Could you check a few things on this model? Use its own coordinates, in mm. A direction names the side the tool comes from. Round coordinates to 2 decimals unless told otherwise and drop trailing zeros. Loops run counter-clockwise (first coordinate to the right, second up) from the corner with the lowest first, then second, coordinate; pieces in that order, holes last. Notation, with made-up numbers: (23.25, -6.75) -> (58.25, -6.75) arc R24 ccw to (58.25, 22.25) -> close; hole circle Ø3 at (-27, -7). An arc over 180 degrees is marked (long way). One line per item, written item: value.
```python
from build123d import *

# Parameters (mm, degrees)
EXTRUDE_1_DEPTH          = 52
FILLET_1_R               = 5
CUT_EXTRUDE_1_DEPTH      = 10
CUT_EXTRUDE_1_DEPTH_BACK = 10
SKETCH_2_R               = 1.5
CUT_EXTRUDE_2_DEPTH      = 10
CUT_EXTRUDE_2_DEPTH_BACK = 1.5


with BuildPart() as part:
    # Эскиз1 → Бобышка-Вытянуть1 (new body)
    with BuildSketch(Plane(origin=(0, 0, 0), x_dir=(1, 0, 0), z_dir=(0, 1, 0))):
        Polygon((-17.5, -4.485282754), (-17.5, -8.485282754), (-6, -8.485282754), (-6, 4.485282754), (6, 4.485282754), (6, -8.485282754), (17.5, -8.485282754), (17.5, -4.485282754), (10, -4.485282754), (10, 8.485282754), (-10, 8.485282754), (-10, -4.485282754), align=None)
    extrude(amount=EXTRUDE_1_DEPTH)

    # Скругление1
    fillet_1_edges = [part.edges().sort_by_distance(p)[0] for p in [
        (-10, 26, 4.485282754),
        (-10, 26, -8.485282754),
        (10, 26, -8.485282754),
        (10, 26, 4.485282754),
    ]]
    fillet(fillet_1_edges, radius=FILLET_1_R)

    # Эскиз2 → Вырез-Вытянуть1 (cut, two sides: drawn at the far end of the back side and taken through both)
    with BuildSketch(Plane(origin=(0, 0, 4.485282754), x_dir=(-1, 0, 0), z_dir=(0, 0, -1)).offset(-CUT_EXTRUDE_1_DEPTH_BACK)):
        with Locations(Location((13.75, 41.6, 0), (0, 0, 33.557309762))):
            Circle(SKETCH_2_R)
        with Locations(Location((13.75, 31.6, 0), (0, 0, 33.557309762))):
            Circle(SKETCH_2_R)
        with Locations(Location((13.75, 21.6, 0), (0, 0, 33.557309762))):
            Circle(SKETCH_2_R)
        with Locations(Location((13.75, 11.6, 0), (0, 0, 33.557309762))):
            Circle(SKETCH_2_R)
        with Locations(Location((-13.75, 41.6, 0), (0, 0, 213.557309762))):
            Circle(SKETCH_2_R)
        with Locations(Location((-13.75, 31.6, 0), (0, 0, 146.442690238))):
            Circle(SKETCH_2_R)
        with Locations(Location((-13.75, 21.6, 0), (0, 0, 146.442690238))):
            Circle(SKETCH_2_R)
        with Locations(Location((-13.75, 11.6, 0), (0, 0, 146.442690238))):
            Circle(SKETCH_2_R)
    extrude(amount=CUT_EXTRUDE_1_DEPTH + CUT_EXTRUDE_1_DEPTH_BACK, mode=Mode.SUBTRACT)

    # Эскиз3 → Вырез-Вытянуть2 (cut, two sides: drawn at the far end of the back side and taken through both)
    with BuildSketch(Plane(origin=(0, 0, 4.485282754), x_dir=(-1, 0, 0), z_dir=(0, 0, -1)).offset(-CUT_EXTRUDE_2_DEPTH_BACK)):
        Polygon((13.75, 38.424573519), (16.5, 40.01228676), (16.5, 43.18771324), (13.75, 44.775426481), (11, 43.18771324), (11, 40.01228676), align=None)
        Polygon((-11, 40.01228676), (-13.75, 38.424573519), (-16.5, 40.01228676), (-16.5, 43.18771324), (-13.75, 44.775426481), (-11, 43.18771324), align=None)
        Polygon((13.75, 28.424573519), (16.5, 30.01228676), (16.5, 33.18771324), (13.75, 34.775426481), (11, 33.18771324), (11, 30.01228676), align=None)
        Polygon((-11, 30.01228676), (-13.75, 28.424573519), (-16.5, 30.01228676), (-16.5, 33.18771324), (-13.75, 34.775426481), (-11, 33.18771324), align=None)
        Polygon((13.75, 18.424573519), (16.5, 20.01228676), (16.5, 23.18771324), (13.75, 24.775426481), (11, 23.18771324), (11, 20.01228676), align=None)
        Polygon((-11, 20.01228676), (-13.75, 18.424573519), (-16.5, 20.01228676), (-16.5, 23.18771324), (-13.75, 24.775426481), (-11, 23.18771324), align=None)
        Polygon((13.75, 8.424573519), (16.5, 10.01228676), (16.5, 13.18771324), (13.75, 14.775426481), (11, 13.18771324), (11, 10.01228676), align=None)
        Polygon((-11, 10.01228676), (-13.75, 8.424573519), (-16.5, 10.01228676), (-16.5, 13.18771324), (-13.75, 14.775426481), (-11, 13.18771324), align=None)
    extrude(amount=CUT_EXTRUDE_2_DEPTH + CUT_EXTRUDE_2_DEPTH_BACK, mode=Mode.SUBTRACT)


solid = part.part
```
(1) We'd pull the mould along Y, two halves only. Please class faces 3 (the face through (-11, 42, 4)), 4 (the face through (-10, 26, -2)), 5 (the face through (0, 0, -6)), 6 (the face through (-13, 30, 5.985)): +Y half, -Y half, draft (parallel to the pull), parting line (faces both ways), or undercut.
Results below:
face 3: undercut
face 4: draft
face 5: -Y half
face 6: undercut
(2) Imagine slicing it at A-A on y = 41.6. Give the number of separate pieces and of enclosed holes in the cut face, then the cut area to 3 significant figures.
Results below:
separate pieces: 3
enclosed holes: 0
area: 207 mm²
(3) Imagine slicing it at B-B on y = 5. Write out the boundary of the cut face in (x, z).
Results below:
outline: (-17.5, 4.49) -> (-15, 4.49) arc R5 cw to (-10, -0.51) -> (-10, -3.49) arc R5 ccw to (-5, -8.49) -> (5, -8.49) arc R5 ccw to (10, -3.49) -> (10, -0.51) arc R5 cw to (15, 4.49) -> (17.5, 4.49) -> (17.5, 8.49) -> (6, 8.49) -> (6, -4.49) -> (-6, -4.49) -> (-6, 8.49) -> (-17.5, 8.49) -> close
(4) Imagine slicing it at C-C on x = 3. Write out the boundary of the cut face in (y, z), then the cut area to 3 significant figures.
Results below:
outline: (0, -8.49) -> (52, -8.49) -> (52, -4.49) -> (0, -4.49) -> close
area: 208 mm²
(5) Imagine slicing it at D-D on z = -6.75. Write out the boundary of the cut face in (x, y).
Results below:
outline: (-8.79, 0) -> (8.79, 0) -> (8.79, 52) -> (-8.79, 52) -> close
(6) On a 3-axis mill with a long thin cutter (end or side, diameter ignored), from which of +Z, -Z, +X, -X, +Y, -Y can I reach the whole of each face in a straight line? I mean faces 1 (the face through (12.089, 13.816, 4.649)), 2 (the face through (-12.765, 32.731, 7.253)). Say none if no direction works.
Results below:
face 1: -Z
face 2: +Z, -Z
(7) For pin 1 Ø3 at (x, y) = (13.5, 20) entering from -Z; pin 2 Ø3.5 at (y, z) = (30, -2) entering from +X; pin 3 Ø6 at (y, z) = (8, 0) entering from -X, each with a flat end and sliding along its axis, tell me the tip position at first contact or that it passes through.
Results below:
pin 1: stops at z = 3.59
pin 2: stops at x = 10.01
pin 3: stops at x = -11.44
(8) Please list where these lines run through material, in increasing order: L1, parallel to Y at x = 13.75, z = 7.9; L2, parallel to X at y = 41.6, z = 7.05; L3, parallel to X at y = 17, z = -2.75.
Results below:
L1: y = 0 to 10.1, 13.1 to 20.1, 23.1 to 30.1, 33.1 to 40.1, 43.1 to 52
L2: x = -17.5 to -15.25, -12.25 to -6, 6 to 12.25, 15.25 to 17.5
L3: x = -10 to -6, 6 to 10
